Read the model definition and answer for the solid it produces. Units are mm, in the model's axes. A direction names the side the tool comes from. Coordinates: 2 decimals unless noted, no trailing zeros. Order: outer loops, then holes, each group sorted by start corner. A loop starts at its lowest first (then second) coordinate and runs counter-clockwise, first axis right, second up. Notation, with made-up numbers: (40, -3) - (84, -3) arc R23 ccw to (84, 36) - close; hole circle Ø5 at (84, 4.5). An arc over 180 degrees is marked (long way). Use one line per item in the form item = value.
```python
from build123d import *

# Parameters (mm, degrees)
MODEL_W                 = 25.06
MODEL_H                 = 128.4
MODEL_R                 = 1.25
MODEL_R_2               = 1.45
BOSS_EXTRU_1_DEPTH      = 2.5
CHANFREIN1_SIZE         = 1.4
ESQUISSE1_R             = 1.4
ESQUISSE1_R_2           = 3.5
ESQUISSE1_R_3           = 2
ENL_V_MAT_EXTRU_1_DEPTH = 131.846526893


with BuildPart() as part:
    # Model → Boss.-Extru.1 (new body)
    with BuildSketch(Plane.XY):
        with Locations((12.53, 64.2)):
            Rectangle(MODEL_W, MODEL_H)
        with Locations((2.37, 14.7)):
            Circle(MODEL_R, mode=Mode.SUBTRACT)
        with Locations((12.53, 14.7)):
            Circle(MODEL_R, mode=Mode.SUBTRACT)
        with Locations((7.45, 14.7)):
            Circle(MODEL_R, mode=Mode.SUBTRACT)
        with Locations((7.45, 113.7)):
            Circle(MODEL_R_2, mode=Mode.SUBTRACT)
        with Locations((17.61, 14.7)):
            Circle(MODEL_R, mode=Mode.SUBTRACT)
        with BuildLine():
            Line((9.895403852, 123.75), (5.004596148, 123.75))
            ThreePointArc((5.004596148, 123.75), (4.5, 125.4), (5.004596148, 127.05))
            Line((5.004596148, 127.05), (9.895403852, 127.05))
            ThreePointArc((9.895403852, 127.05), (10.4, 125.4), (9.895403852, 123.75))
        make_face(mode=Mode.SUBTRACT)
        with BuildLine():
            Line((9.895403852, 1.35), (5.004596148, 1.35))
            ThreePointArc((5.004596148, 1.35), (4.5, 3), (5.004596148, 4.65))
            Line((5.004596148, 4.65), (9.895403852, 4.65))
            ThreePointArc((9.895403852, 4.65), (10.4, 3), (9.895403852, 1.35))
        make_face(mode=Mode.SUBTRACT)
    extrude(amount=BOSS_EXTRU_1_DEPTH)

    # Chanfrein1
    chanfrein1_edges = [part.edges().sort_by_distance(p)[0] for p in [
        (6, 113.7, 2.5),
    ]]
    chamfer(chanfrein1_edges, length=CHANFREIN1_SIZE)

    # Esquisse1 → Enlèv. mat.-Extru.1 (cut, through all)
    with BuildSketch(Plane.XY.offset(2.5)):
        with Locations((18.81464069, 99.211522536)):
            Circle(ESQUISSE1_R)
        with Locations((18.826761896, 87.211528658)):
            Circle(ESQUISSE1_R)
        with Locations((18.838883102, 75.21153478)):
            Circle(ESQUISSE1_R)
        with Locations((18.851004308, 63.211540902)):
            Circle(ESQUISSE1_R)
        with Locations((18.863125514, 51.211547023)):
            Circle(ESQUISSE1_R)
        with Locations((18.875246719, 39.211553145)):
            Circle(ESQUISSE1_R)
        with Locations((18.887367925, 27.211559267)):
            Circle(ESQUISSE1_R)
        with Locations((10.16464508, 99.202785174)):
            Circle(ESQUISSE1_R_2)
        with Locations((10.176766286, 87.202791295)):
            Circle(ESQUISSE1_R_2)
        with Locations((10.188887492, 75.202797417)):
            Circle(ESQUISSE1_R_2)
        with Locations((10.201008698, 63.202803539)):
            Circle(ESQUISSE1_R_2)
        with Locations((10.213129904, 51.202809661)):
            Circle(ESQUISSE1_R_2)
        with Locations((10.225251109, 39.202815783)):
            Circle(ESQUISSE1_R_2)
        with Locations((7.900573508, 27.200461502)):
            Circle(ESQUISSE1_R_3)
    extrude(amount=-ENL_V_MAT_EXTRU_1_DEPTH, mode=Mode.SUBTRACT)


solid = part.part
```
(1) Straight lines are drawn through the part: L1, parallel to X at y = 27, z = 1.85; L2, parallel to Y at x = 5.5, z = 0.8; L3, parallel to X at y = 15.5, z = 0.85. For each, find the intervals that lie inside material, in ascending order.
Answer list:
L1 = 0 to 5.91, 9.89 to 17.5, 20.27 to 25.06
L2 = 0 to 1.35, 4.65 to 123.75, 127.05 to 128.4
L3 = 0 to 1.41, 3.33 to 6.49, 8.41 to 11.57, 13.49 to 16.65, 18.57 to 25.06
(2) Section B-B, the plane y = 14.7 is taken. Write down the section's boundary in (x, z).
Answer list:
outline = (0, 0) - (1.12, 0) - (1.12, 2.5) - (0, 2.5) - close; (3.62, 0) - (6.2, 0) - (6.2, 2.5) - (3.62, 2.5) - close; (8.7, 0) - (11.28, 0) - (11.28, 2.5) - (8.7, 2.5) - close; (13.78, 0) - (16.36, 0) - (16.36, 2.5) - (13.78, 2.5) - close; (18.86, 0) - (25.06, 0) - (25.06, 2.5) - (18.86, 2.5) - close
(3) Section C-C, the plane z = 1.5 is taken. State how many separate pieces and enclosed holes the cut face has, then the cut area to 3 significant figures.
Answer list:
separate_pieces = 1
enclosed_holes = 21
area = 2,860 mm2
(4) The mould has two halves that part along Y. Classify faces 3 (the cylindrical face through (17.45, 15.94, 1.23)), 4 (the flat face through (12, 0, 1)), 5 (the flat face through (25.06, 63, 1)): +Y half, -Y half, draft (parallel to the pull), parting line (faces both ways), or undercut.
Answer list:
face_3 = undercut
face_4 = -Y half
face_5 = draft
(5) Section A-A, the plane x = 2.37 is taken. Write down the section's boundary in (y, z).
Answer list:
outline = (0, 0) - (13.45, 0) - (13.45, 2.5) - (0, 2.5) - close; (15.95, 0) - (128.4, 0) - (128.4, 2.5) - (15.95, 2.5) - close
(6) Which of the six approach directions +Z, -Z, +X, -X, +Y, -Y give full straight-line access (tool end or side, diameter ignored) to faces 1 (the flat face through (7, 123.75, 1)), 2 (the flat face through (0, 63, 1))?
Answer list:
face_1 = +Z, -Z
face_2 = +Z, -Z, -X, +Y, -Y
